from build123d import *

# Parameters (mm, degrees)
F0_W     = 18.034
F0_H     = 38.608
F1_DEPTH = 12.7
F2_R     = 1.27


with BuildPart() as f1:
    # F0 (on Top) → F1 (new body)
    with BuildSketch(Plane.XY):
        Polygon((-1.5875, 14.2875), (-1.5875, -1.5875), (19.6215, -1.5875), (19.6215, 40.1955), (-1.5875, 40.1955), (-1.5875, 26.9875), (-1.5875, 25.4), (-1.5875, 15.875), align=None)
        with Locations((9.017, 19.304)):
            Rectangle(F0_W, F0_H, mode=Mode.SUBTRACT)
        with BuildLine():
            Line((-6.35, 14.2875), (-1.5875, 14.2875))
            Line((-1.5875, 14.2875), (-1.5875, 15.875))
            Line((-1.5875, 15.875), (-6.35, 15.875))
            ThreePointArc((-6.35, 15.875), (-11.1125, 20.6375), (-6.35, 25.4))
            Line((-6.35, 25.4), (-1.5875, 25.4))
            Line((-1.5875, 25.4), (-1.5875, 26.9875))
            Line((-1.5875, 26.9875), (-6.35, 26.9875))
            ThreePointArc((-6.35, 26.9875), (-12.7, 20.6375), (-6.35, 14.2875))
        make_face()
    extrude(amount=F1_DEPTH)

    # F2
    f2_edges = [f1.edges().sort_by_distance(p)[0] for p in [
        (19.6215, -1.5875, 6.35),
        (-1.5875, -1.5875, 6.35),
        (-1.5875, 40.1955, 6.35),
        (19.6215, 40.1955, 6.35),
    ]]
    fillet(f2_edges, radius=F2_R)


solid = f1.part
The model under review builds one solid part; all positions refer to its coordinate system, in mm. A direction names the side the tool comes from. Give positions to 0.01 mm unless a question says otherwise; leave off trailing zeros. Order: outer loops, then holes, each group sorted by start corner. A loop starts at its lowest first (then second) coordinate and runs counter-clockwise, first axis right, second up. Notation, with made-up numbers: M 74.25,44.5 L 101.25,44.5 A27 cw 101.25,68.5 Z; hole C 68,46 d1. An arc over 180 degrees is marked long. Answer in a Markdown table with one row per item. Add a question column.
1. Add section C-C on y = 35. State the section outline as (x, z) points.
2. For pin 1 Ø1.4 at (x, z) = (-4, 6) entering from -Y; pin 2 Ø1.5 at (y, z) = (16.5, 2) entering from -X; pin 3 Ø3.5 at (y, z) = (32, 4.5) entering from -X, all flat-tipped, find the tip position at first contact; note any pin that passes through.
3. Machinability: for faces 1 (the flat face through (9, 40.196, 6)), 2 (the flat face through (-4, 14.288, 6)), 3 (the flat face through (19.622, 19, 6)), 4 (the flat face through (9, 38.608, 6)), 5 (the flat face through (-4, 26.988, 6)), which of the approach directions +Z, -Z, +X, -X, +Y, -Y give a long, thin tool a straight path to every point of the face, cutting with its end or side? Answer none if there is none.
4. Mouldability with a two-part tool opening along X and no side actions: class faces 6 (the flat face through (0, 19, 6)), 7 (the flat face through (-0.2, 19.4, 0)), 8 (the cylindrical face through (19.259, 39.814, 6.439)), 9 (the flat face through (-1.588, 33, 6)) as released by +X, released by -X, zero draft, split by the parting line, or undercut.
5. To check wall thickness, follow line 1 along X through (y, z) = (36, 11.5); line 2 along Y through (x, z) = (7.5, 8.75); line 3 along X through (y, z) = (22.5, 6.25). State the ranges of each line that lie inside material, in increasing order.
6. Add section B-B on z = 7.5. Count the separate pieces of the cut face and the enclosed holes in it, plus the area to 3 significant figures.
7. Add section A-A on x = -3.5. State the section outline as (y, z) points (1 decimal).
8. Add section D-D on y = 20. State the section outline as (x, z) points, plus the area to 3 significant figures.
The answers:
| question | item | result |
|---|---|---|
| 1 | outline | M -1.59,0 L 0,0 L 0,12.7 L -1.59,12.7 Z; M 18.03,0 L 19.62,0 L 19.62,12.7 L 18.03,12.7 Z |
| 2 | pin 1 | y = 14.29 |
| 2 | pin 2 | x = -11.72 |
| 2 | pin 3 | x = -1.59 |
| 3 | face 1 | +Z, -Z, +X, -X, +Y |
| 3 | face 2 | +Z, -Z, -X, -Y |
| 3 | face 3 | +Z, -Z, +X, +Y, -Y |
| 3 | face 4 | +Z, -Z |
| 3 | face 5 | +Z, -Z, -X, +Y |
| 4 | face 6 | undercut |
| 4 | face 7 | zero draft |
| 4 | face 8 | released by +X |
| 4 | face 9 | released by -X |
| 5 | line 1 | -1.59 to 0, 18.03 to 19.62 |
| 5 | line 2 | -1.59 to 0, 38.61 to 40.2 |
| 5 | line 3 | -12.42 to -10.73, -1.59 to 0, 18.03 to 19.62 |
| 6 | separate pieces | 1 |
| 6 | enclosed holes | 2 |
| 6 | area | 231 mm2 |
| 7 | outline | M 14.3,0 L 15.9,0 L 15.9,12.7 L 14.3,12.7 Z; M 25.4,0 L 27,0 L 27,12.7 L 25.4,12.7 Z |
| 8 | outline | M -12.67,0 L -11.07,0 L -11.07,12.7 L -12.67,12.7 Z; M -1.59,0 L 0,0 L 0,12.7 L -1.59,12.7 Z; M 18.03,0 L 19.62,0 L 19.62,12.7 L 18.03,12.7 Z |
| 8 | area | 60.6 mm2 |
